Model file for the job. Use its own axes, mm. A direction names the side the tool comes from. Coordinates: 2 decimals unless noted, no trailing zeros. Write each loop counter-clockwise with the first axis right and the second up, starting at its lowest first coordinate (ties: lowest second). Pieces come first, ordered by that corner, then holes.
Q1. Band-saw the part on C-C, the plane z = 16. Write the cut outline in (x, y).
Q2. Band-saw the part on D-D, the plane z = -60. Write the cut outline in (x, y).
Q3. Drill centre lines: probe 1 along Z at (x, y) = (0, 11); probe 2 along Y at (x, z) = (0, -75); probe 3 along Y at (x, z) = (0, 15.5). Where is each one in solid material? Low to high.
Q4. Pull direction X, two halves, no side cores. Call faces 4 (the flat face through (3, -9.5, 109)), 5 (the cylindrical face through (-2.298, -10.91, 60.101)): released by +X, released by -X, zero draft, split by the parting line, or undercut.
Q5. Band-saw the part on A-A, the plane y = 0. Write the cut outline in (x, z), plus the area to 3 significant figures.
Q6. Pin check, flat tips, straight feed: P1, Ø2.5, axis at y = -14, z = 60.5, coming from the -X side; P2, Ø4, axis at x = 13, z = 61, coming from the +Y side; P3, Ø1, axis at x = -13, z = -84, coming from the +Y side; P4, Ø9, axis at x = 0, z = -98.5, coming from the -Y side. Stop position of each tip, or through.
Q7. Which spindle directions (+Z, -Z, +X, -X, +Y, -Y) get a long thin tool onto all of the face, cutting with end or side? Do faces 1 (the cylindrical face through (5.19, -9.98, -0.39)), 2 (the cylindrical face through (-0.499, 13.377, -62.245)), 3 (the flat face through (2.049, -15.035, 103.484)). Say none if no direction does.
Q8. Band-saw the part on B-B, the plane z = 100. Write the cut outline in (x, y), plus the area to 3 significant figures.
from build123d import *

# Parameters (mm, degrees)
SKETCH002_R          = 17.5
SKETCH002_R_2        = 9.65
PAD001_DEPTH         = 109
PAD001_DEPTH_BACK    = 109
SKETCH003_R          = 11.25
SKETCH003_R_2        = 6
POCKET001_DEPTH      = 28
POCKET001_DEPTH_BACK = 28
POCKET002_DEPTH      = 5
SKETCH005_R          = 2.3
POCKET003_DEPTH      = 50
POCKET003_DEPTH_BACK = 50
FILLET001_R          = 3


with BuildPart() as part:
    # Sketch002 → Pad001 (new body, two sides)
    with BuildSketch(Plane.XY) as pad001_sk:
        Circle(SKETCH002_R)
        Circle(SKETCH002_R_2, mode=Mode.SUBTRACT)
    extrude(amount=PAD001_DEPTH)
    extrude(pad001_sk.sketch, amount=-PAD001_DEPTH_BACK)

    # Sketch003 → Pocket001 (cut, two sides)
    with BuildSketch(Plane.XY) as pocket001_sk:
        Circle(SKETCH003_R)
        Circle(SKETCH003_R_2, mode=Mode.SUBTRACT)
    extrude(amount=-POCKET001_DEPTH, mode=Mode.SUBTRACT)
    extrude(pocket001_sk.sketch, amount=POCKET001_DEPTH_BACK, mode=Mode.SUBTRACT)

    # Sketch004 (on DatumPlane) → Pocket002 (cut)
    with BuildSketch(Plane.XZ.offset(17.5)):
        Polygon((0, 95.333333), (4.041452, 97.666667), (4.041452, 102.333333), (0, 104.666667), (-4.041452, 102.333333), (-4.041452, 97.666667), align=None)
        Polygon((4.041452, 57.666667), (4.041452, 62.333333), (0, 64.666667), (-4.041452, 62.333333), (-4.041452, 57.666667), (0, 55.333333), align=None)
        Polygon((0, -64.041452), (3.5, -62.020726), (3.5, -57.979274), (0, -55.958548), (-3.5, -57.979274), (-3.5, -62.020726), align=None)
        Polygon((4.041452, -102.333333), (4.041452, -97.666667), (0, -95.333333), (-4.041452, -97.666667), (-4.041452, -102.333333), (0, -104.666667), align=None)
    extrude(amount=-POCKET002_DEPTH, mode=Mode.SUBTRACT)

    # Sketch005 → Pocket003 (cut, two sides)
    with BuildSketch(Plane.XZ) as pocket003_sk:
        with Locations((0, 60)):
            Circle(SKETCH005_R)
        with Locations((0, 100)):
            Circle(SKETCH005_R)
        with Locations((0, -60)):
            Circle(SKETCH005_R)
        with Locations((0, -100)):
            Circle(SKETCH005_R)
    extrude(amount=-POCKET003_DEPTH, mode=Mode.SUBTRACT)
    extrude(pocket003_sk.sketch, amount=POCKET003_DEPTH_BACK, mode=Mode.SUBTRACT)

    # Fillet001
    fillet001_edges = [part.edges().sort_by_distance(p)[0] for p in [
        (-17.5, 0, 109),
        (-17.5, 0, -109),
    ]]
    fillet(fillet001_edges, radius=FILLET001_R)


solid = part.part
Answer sheet:
1. outline: circle Ø35 at (0, 0); hole circle Ø22.5 at (0, 0)
2. outline: (-3.5, -17.15) - (-3.5, -12.5) - (-2.3, -12.5) - (-2.3, -9.37) arc R9.65 cw to (-2.3, 9.37) - (-2.3, 17.35) arc R17.5 ccw to start; (2.3, -12.5) - (3.5, -12.5) - (3.5, -17.15) arc R17.5 ccw to (2.3, 17.35) - (2.3, 9.37) arc R9.65 cw to (2.3, -9.37) - close
3. probe 1: z = -109 to -102.3, -97.7 to -62.3, -57.7 to -28, 28 to 57.7, 62.3 to 97.7, 102.3 to 109
3. probe 2: y = -17.5 to -9.65, 9.65 to 17.5
3. probe 3: y = -17.5 to -11.25, 11.25 to 17.5
4. face 4: zero draft
4. face 5: undercut
5. outline: (-17.5, -106) arc R3 ccw to (-14.5, -109) - (-9.65, -109) - (-9.65, -28) - (-11.25, -28) - (-11.25, 28) - (-9.65, 28) - (-9.65, 109) - (-14.5, 109) arc R3 ccw to (-17.5, 106) - close; (9.65, -109) - (14.5, -109) arc R3 ccw to (17.5, -106) - (17.5, 106) arc R3 ccw to (14.5, 109) - (9.65, 109) - (9.65, 28) - (11.25, 28) - (11.25, -28) - (9.65, -28) - close
5. area: 3,240 mm2
6. P1: stops at x = -11.99
6. P2: stops at y = 13.61
6. P3: stops at y = 12.25
6. P4: stops at y = -17.5
7. face 1: none
7. face 2: +Y, -Y
7. face 3: -Y
8. outline: (-4.04, -17.03) - (-4.04, -12.5) - (-2.3, -12.5) - (-2.3, -9.37) arc R9.65 cw to (-2.3, 9.37) - (-2.3, 17.35) arc R17.5 ccw to start; (2.3, -12.5) - (4.04, -12.5) - (4.04, -17.03) arc R17.5 ccw to (2.3, 17.35) - (2.3, 9.37) arc R9.65 cw to (2.3, -9.37) - close
8. area: 581 mm2
